Build history of the part. All positions in model axes, mm. Round coordinates to 2 decimals unless told otherwise and drop trailing zeros. Order: outer loops, then holes, each group sorted by start corner. A loop starts at its lowest first (then second) coordinate and runs counter-clockwise, first axis right, second up. Notation, with made-up numbers: (0.25, 6.5) -> (29.25, 6.5) arc R21 cw to (29.25, 31.5) -> close; hole circle Ø10 at (56.5, -3.5). An arc over 180 degrees is marked (long way). Write item = value, one per line.
from build123d import *

# Parameters (mm, degrees)
SKETCH1_R             = 161.157000012
SKETCH1_R_2           = 148.457000012
SKETCH1_R_3           = 2.38125
BOSS_EXTRUDE1_DEPTH   = 10
CHAMFER1_SIZE         = 0.889
CHAMFER2_SIZE         = 2.54
CHAMFER2_SIZE2        = 2.131313063
CHAMFER2_PART_2_SIZE  = 2.54
CHAMFER2_PART_2_SIZE2 = 2.131313063
CHAMFER2_PART_3_SIZE  = 2.54
CHAMFER2_PART_3_SIZE2 = 2.131313063


with BuildPart() as part:
    # Sketch1 → Boss-Extrude1 (new body)
    with BuildSketch(Plane(origin=(0, 0, 0), x_dir=(1, 0, 0), z_dir=(0, 1, 0))):
        Circle(SKETCH1_R)
        Circle(SKETCH1_R_2, mode=Mode.SUBTRACT)
        with Locations((0, 154.5)):
            Circle(SKETCH1_R_3, mode=Mode.SUBTRACT)
        with Locations((133.800924885, 77.25)):
            Circle(SKETCH1_R_3, mode=Mode.SUBTRACT)
        with Locations((133.800924885, -77.25)):
            Circle(SKETCH1_R_3, mode=Mode.SUBTRACT)
        with Locations((0, -154.5)):
            Circle(SKETCH1_R_3, mode=Mode.SUBTRACT)
        with Locations((-133.800924885, -77.25)):
            Circle(SKETCH1_R_3, mode=Mode.SUBTRACT)
        with Locations((-133.800924885, 77.25)):
            Circle(SKETCH1_R_3, mode=Mode.SUBTRACT)
    extrude(amount=BOSS_EXTRUDE1_DEPTH)

    # Chamfer1
    chamfer1_edges = [part.edges().sort_by_distance(p)[0] for p in [
        (-161.157000012, 0, 0),
        (-161.157000012, 10, 0),
        (-148.457000012, 0, 0),
        (-148.457000012, 10, 0),
    ]]
    chamfer(chamfer1_edges, length=CHAMFER1_SIZE)

    # Chamfer2
    chamfer2_edges = [part.edges().sort_by_distance(p)[0] for p in [
        (131.419674885, 0, 77.25),
    ]]
    chamfer2_side = [part.faces().sort_by_distance(p)[0] for p in [
        (-155.734936427, 0, 0),
    ]]
    chamfer(chamfer2_edges, length=CHAMFER2_SIZE, length2=CHAMFER2_SIZE2, reference=chamfer2_side[0])

    # Chamfer2 part 2
    chamfer2_part_2_edges = [part.edges().sort_by_distance(p)[0] for p in [
        (-136.182174885, 0, 77.25),
    ]]
    chamfer2_part_2_side = [part.faces().sort_by_distance(p)[0] for p in [
        (-136.182174885, 5, 77.25),
    ]]
    chamfer(chamfer2_part_2_edges, length=CHAMFER2_PART_2_SIZE, length2=CHAMFER2_PART_2_SIZE2, reference=chamfer2_part_2_side[0])

    # Chamfer2 part 3
    chamfer2_part_3_edges = [part.edges().sort_by_distance(p)[0] for p in [
        (-2.38125, 0, -154.5),
    ]]
    chamfer2_part_3_side = [part.faces().sort_by_distance(p)[0] for p in [
        (-2.38125, 5, -154.5),
    ]]
    chamfer(chamfer2_part_3_edges, length=CHAMFER2_PART_3_SIZE, length2=CHAMFER2_PART_3_SIZE2, reference=chamfer2_part_3_side[0])


solid = part.part
Q1. Cut at A-A, the plane z = 0. List the corners of the cut face in (x, y), and give its area (3 significant figures).
Check values:
outline = (-161.16, 0.89) -> (-160.27, 0) -> (-149.35, 0) -> (-148.46, 0.89) -> (-148.46, 9.11) -> (-149.35, 10) -> (-160.27, 10) -> (-161.16, 9.11) -> close; (148.46, 0.89) -> (149.35, 0) -> (160.27, 0) -> (161.16, 0.89) -> (161.16, 9.11) -> (160.27, 10) -> (149.35, 10) -> (148.46, 9.11) -> close
area = 251 mm²
Q2. Flat gauge pins, fed straight in: pin 1 (3 mm diameter, centred on x = 133.8, z = 77.25, fed in from +Y); pin 2 (5.5 mm diameter, centred on x = -133.8, z = 77.25, fed in from -Y); pin 3 (3 mm diameter, centred on x = -58.5, y = 3.5, fed in from +Z); pin 4 (1 mm diameter, centred on x = -17, y = 1.5, fed in from -Z). Where does each tip first touch, or does it go through?
Check values:
pin_1 = through
pin_2 = 2.1
pin_3 = 150.74
pin_4 = -160.31
Q3. Probe probe 1 along Z at (x, y) = (0, 8.5); probe 2 along X at (y, z) = (3, -77.25); probe 3 along X at (y, z) = (4.5, -2). List the from-to ranges inside material, lowest first.
Check values:
probe_1 = -161.16 to -156.88, -152.12 to -148.46, 148.46 to 152.12, 156.88 to 161.16
probe_2 = -141.44 to -136.18, -131.42 to -126.78, 126.78 to 131.42, 136.18 to 141.44
probe_3 = -161.14 to -148.44, 148.44 to 161.14
Q4. Mould opens along Z. For faces 1 (the face through (-131.478, 2.381, 78.213)), 2 (the face through (-34.936, 4.942, 157.325)), 3 (the face through (-131.3, 0, -72)) say: released by +Z, released by -Z, zero draft, split by the parting line, or undercut.
Check values:
face_1 = undercut
face_2 = split by the parting line
face_3 = zero draft
